Autodesk Inventor part; units mm, degrees
ref_plane "YZ Plane" through (0, 0, 0) normal (1, 0, 0) x (0, 1, 0)
ref_plane "XZ Plane" through (0, 0, 0) normal (0, 1, 0) x (-1, 0, 0)
ref_plane "XY Plane" through (0, 0, 0) normal (0, 0, 1) x (1, 0, 0)
sketch "Esboço1" plane through (0, 0, 0) normal (0, 1, 0) x (-1, 0, 0)
  line L0 (148.75, 5) -> (-148.75, 5)
  line L1 (-148.75, 5) -> (-148.75, -5)
  line L2 (-148.75, -5) -> (148.75, -5)
  line L3 (148.75, -5) -> (148.75, 5)
  line L4 (148.75, 5) -> (-148.75, -5) construction
  line L5 (-148.75, 5) -> (148.75, -5) construction
  point P0 (0, 0)
  dimension "d0" = 297.5
  dimension "d1" = 10
extrude "Placa1" add sketch "Esboço1" along normal blind 0.5
sketch "Esboço2" plane through (0, 0, 0) normal (0, -1, 0) x (1, 0, 0)
  line L0 (-148.75, -5) -> (-148.75, 5)
  line L1 (148.75, -5) -> (-148.75, -5)
  line L2 (148.75, 5) -> (148.75, -5)
  point P0 (0, 0)
  point P1 (-98.75, -1)
  point P2 (98.75, -1)
  dimension "d3" = 50
  dimension "d4" = 4
  dimension "d5" = 4
  dimension "d6" = 50
hole "Furo1" at (-98.75, 0, -1) at (98.75, 0, -1) direction (0, 1, 0) diameter 3 end through all
equation "\"d12\" = Espessura"
equation "\"d2\" = Espessura"
equation "\"Raio_vergadura\" = Espessura"
equation "\"Largura_alívio_de_vergadura\" = Espessura"
equation "\"Profundidade_alívio_de_vergadura\" = 0.5 * Espessura"
equation "\"Tamanho_alívio_de_dobra\" = 4 * Espessura"
equation "\"Remanescente_mínimo\" = 2 * Espessura"
equation "\"Raiodetransição\" = Raio_vergadura"
equation "\"Tamanho_de_raio_de_Jacobi\" = Raio_vergadura"
equation "\"TamanhoFolga\" = Espessura"
properties part number "Lateral 1 Gaveta" material "PMMA plástico"
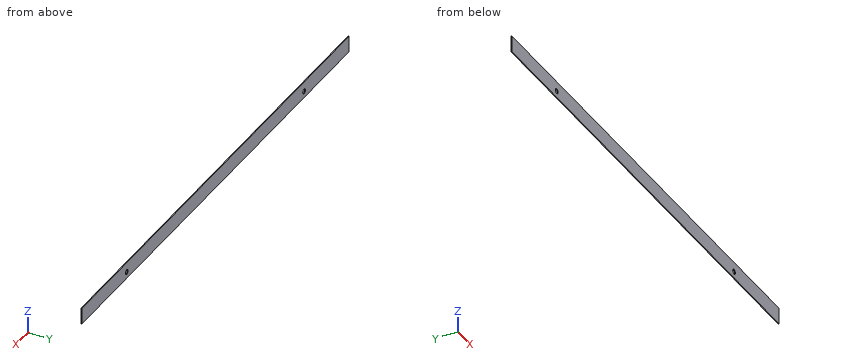
Input: part model. Units: mm. Frame: model coordinates. Coordinates: 2 decimals unless noted, no trailing zeros. Loops run counter-clockwise (first coordinate to the right, second up) from the corner with the lowest first, then second, coordinate; pieces in that order, holes last. Notation, with made-up numbers: (2, 84) - (16, 84) arc R17 ccw to (16, 112) - close; hole circle Ø8 at (34, -28). An arc over 180 degrees is marked (long way). Answer in a Markdown table with one row per item. Add a question column.
Item 1: Section query A-A on z = -1. Return the cut outline in (x, y), then the cut area to 3 significant figures.
Item 2: Line query: line 1 along X through (y, z) = (0.35, -1); line 2 along Z through (x, y) = (-98.75, 0.35); line 3 along X through (y, z) = (0.2, 0). Output: solid intervals per line, ascending. Write a range as [from, to].
Item 3: Contact query for a flat-ended pin moving along its axis: P1, Ø2.5, axis at x = -98.75, z = -1, coming from the -Y side. Output: stop coordinate, or through.
Recorded:
| question | item | result |
|---|---|---|
| 1 | outline | (-148.75, 0) - (-100.25, 0) - (-100.25, 0.5) - (-148.75, 0.5) - close; (-97.25, 0) - (97.25, 0) - (97.25, 0.5) - (-97.25, 0.5) - close; (100.25, 0) - (148.75, 0) - (148.75, 0.5) - (100.25, 0.5) - close |
| 1 | area | 146 mm^2 |
| 2 | line 1 | [-148.75, -100.25], [-97.25, 97.25], [100.25, 148.75] |
| 2 | line 2 | [-5, -2.5], [0.5, 5] |
| 2 | line 3 | [-148.75, -99.87], [-97.63, 97.63], [99.87, 148.75] |
| 3 | P1 | through |
